Print and shaded views of the part. All mm, measured from the part's lowest x, y and z. Give positions to 0.01 mm unless a question says otherwise; leave off trailing zeros. Loops run counter-clockwise (first coordinate to the right, second up) from the corner with the lowest first, then second, coordinate; pieces in that order, holes last. Notation, with made-up numbers: (-24.75, -1.75) - (30.25, -1.75) arc R18 cw to (30.25, 15.25) - close; hole circle Ø8 at (-27, 57). An arc over 180 degrees is marked (long way). Return JSON: item names as keys, results as strings.
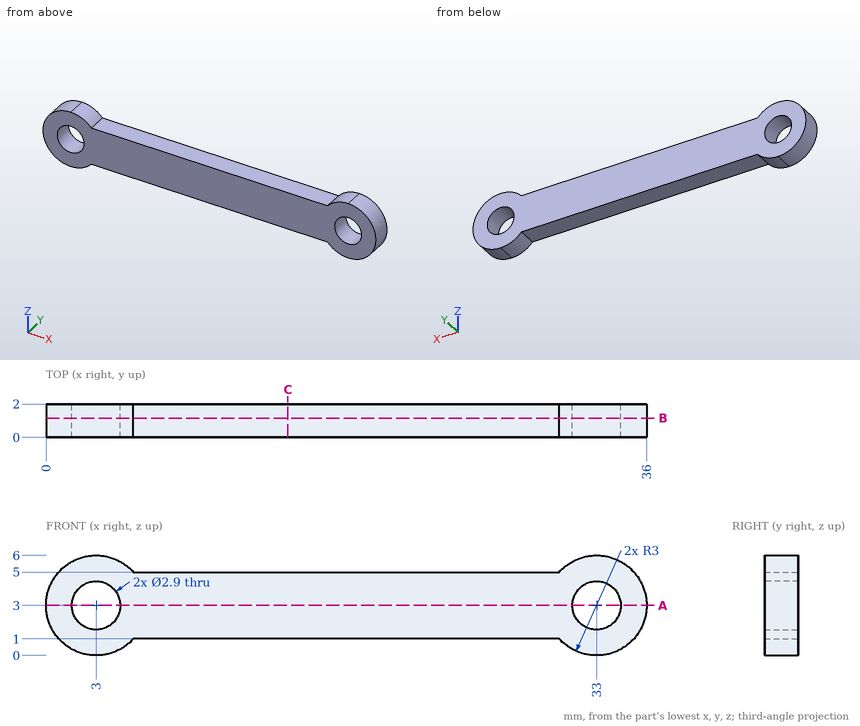
1. Drill centre lines: probe 1 along X at (y, z) = (0.55, 3); probe 2 along Z at (x, y) = (33, 0.65); probe 3 along Z at (x, y) = (26, 1.55). Where is each one in solid material? Low to high.
Values follow:
{"probe 1": "x = 0 to 1.55, 4.45 to 31.55, 34.45 to 36", "probe 2": "z = 0 to 1.55, 4.45 to 6", "probe 3": "z = 1 to 5"}
2. Cut at B-B, the plane y = 1.15. Write the cut outline in (x, z).
Values follow:
{"outline": "(5.24, 1) - (30.76, 1) arc R3 ccw (long way) to (30.76, 5) - (5.24, 5) arc R3 ccw (long way) to start; hole circle Ø2.9 at (3, 3); hole circle Ø2.9 at (33, 3)"}
3. Cut at A-A, the plane z = 3. Write the cut outline in (x, y).
Values follow:
{"outline": "(0, 0) - (1.55, 0) - (1.55, 2) - (0, 2) - close; (4.45, 0) - (31.55, 0) - (31.55, 2) - (4.45, 2) - close; (34.45, 0) - (36, 0) - (36, 2) - (34.45, 2) - close"}
4. Drop flat-ended pins along their axis: P1, Ø2.5, axis at x = 33, z = 3, coming from the +Y side; P2, Ø1, axis at x = 26.5, y = 1, coming from the -Z side. Give the stop position or say it passes through.
Values follow:
{"P1": "passes through", "P2": "stops at z = 1"}
5. Cut at C-C, the plane x = 14.5. Write the cut outline in (y, z), plus the area to 3 significant figures.
Values follow:
{"outline": "(0, 1) - (2, 1) - (2, 5) - (0, 5) - close", "area": "8.00 mm²"}
